Read the model definition and answer for the solid it produces. Units are mm, in the model's axes. A direction names the side the tool comes from. Coordinates: 2 decimals unless noted, no trailing zeros. Loops run counter-clockwise (first coordinate to the right, second up) from the corner with the lowest first, then second, coordinate; pieces in that order, holes last. Notation, with made-up numbers: M 20,49.5 L 35,49.5 A9 cw 35,66.5 Z; hole C 8.25,5.25 d1. An arc over 180 degrees is marked long. Put each result on its own line as item: value.
from build123d import *

# Parameters (mm, degrees)
SKETCH_1_W          = 12
SKETCH_1_H          = 12
SKETCH_1_W_2        = 9
SKETCH_1_H_2        = 9
EXTRUDE_1_DEPTH     = 40
SKETCH_2_R          = 2.6
SKETCH_2_R_2        = 2.1
CUT_EXTRUDE_1_DEPTH = 30


with BuildPart() as part:
    # ｽｹｯﾁ1 → ﾎﾞｽ - 押し出し1 (new body)
    with BuildSketch(Plane.XY):
        Rectangle(SKETCH_1_W, SKETCH_1_H)
        Rectangle(SKETCH_1_W_2, SKETCH_1_H_2, mode=Mode.SUBTRACT)
    extrude(amount=EXTRUDE_1_DEPTH)

    # ｽｹｯﾁ2 → ｶｯﾄ - 押し出し1 (cut)
    with BuildSketch(Plane(origin=(0, 6, 0), x_dir=(1, 0, 0), z_dir=(0, 1, 0))):
        with Locations((0, -5)):
            Circle(SKETCH_2_R)
        with Locations((0, -35)):
            Circle(SKETCH_2_R_2)
    extrude(amount=-CUT_EXTRUDE_1_DEPTH, mode=Mode.SUBTRACT)


solid = part.part
1) Find section A-A, the plane z = 5. Write down the section's boundary in (x, y), plus the area to 3 significant figures.
Answer list:
outline: M -6,-6 L -2.6,-6 L -2.6,-4.5 L -4.5,-4.5 L -4.5,4.5 L -2.6,4.5 L -2.6,6 L -6,6 Z; M 2.6,-6 L 6,-6 L 6,6 L 2.6,6 L 2.6,4.5 L 4.5,4.5 L 4.5,-4.5 L 2.6,-4.5 Z
area: 47.4 mm^2
2) Which of the six approach directions +Z, -Z, +X, -X, +Y, -Y give full straight-line access (tool end or side, diameter ignored) to faces 1 (the flat face through (4.5, 0, 20)), 2 (the cylindrical face through (1.2, 5.26, 7.307))?
Answer list:
face 1: +Z, -Z
face 2: +Y, -Y
3) Determine the mould class of faces 3 (the flat face through (-6, 0, 20)), 4 (the flat face through (0, -4.5, 20)), 5 (the flat face through (5, 0, 40)) for opening direction X: released by +X, released by -X, zero draft, split by the parting line, or undercut.
Answer list:
face 3: released by -X
face 4: undercut
face 5: zero draft
4) Straight lines are drawn through the part: line 1 (Z direction, x = 0, y = -5.1); line 2 (Y direction, x = -2.5, z = 37.5); line 3 (X direction, y = 5.4, z = 5). For each, find the intervals that lie inside material, in ascending order. Write a range as [from, to].
Answer list:
line 1: z = [0, 2.4], [7.6, 32.9], [37.1, 40]
line 2: y = [-6, -4.5], [4.5, 6]
line 3: x = [-6, -2.6], [2.6, 6]
5) Find section D-D, the plane z = 32.5. Write down the section's boundary in (x, y), plus the area to 3 significant figures.
Answer list:
outline: M -6,-6 L 6,-6 L 6,6 L -6,6 Z; hole M -4.5,-4.5 L 4.5,-4.5 L 4.5,4.5 L -4.5,4.5 Z
area: 63.0 mm^2
6) Find section B-B, the plane x = 3.25. Write down the section's boundary in (y, z).
Answer list:
outline: M -6,0 L -4.5,0 L -4.5,40 L -6,40 Z; M 4.5,0 L 6,0 L 6,40 L 4.5,40 Z
